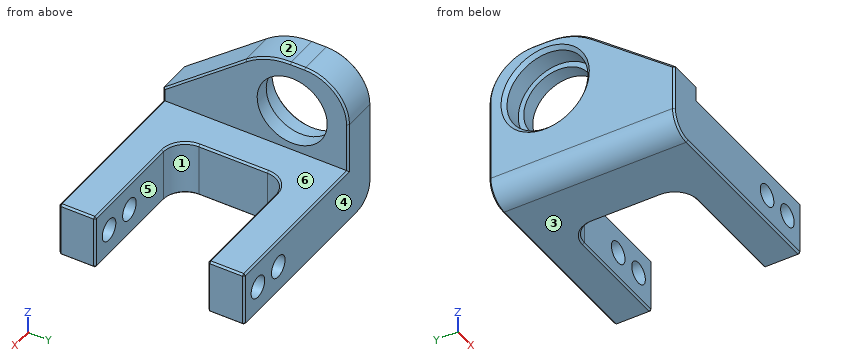
```python
from build123d import *

# Parameters (mm, degrees)
BOSS_EXTRUDE1_DEPTH = 50.8
SKETCH2_R           = 11.1
CUT_EXTRUDE1_DEPTH  = 6
SKETCH4_R           = 9.6
CUT_EXTRUDE2_DEPTH  = 79.563869558
SKETCH5_R           = 3
CUT_EXTRUDE3_DEPTH  = 83.512311809
CUT_EXTRUDE4_DEPTH  = 83.512311809
FILLET3_R           = 20
FILLET4_R           = 12
SKETCH8_W           = 36
SKETCH8_H           = 30.8
CUT_EXTRUDE5_DEPTH  = 80.805586271
CHAMFER2_SIZE       = 1
FILLET6_R           = 6
FILLET5_R           = 6
CHAMFER3_SIZE       = 0.5


with BuildPart() as part:
    # Sketch1 → Boss-Extrude1 (new body)
    with BuildSketch(Plane(origin=(0, 0, 0), x_dir=(1, 0, 0), z_dir=(0, 1, 0))):
        Polygon((-56, 7.5), (-56, -33.04), (-46, -33.04), (-46, -7.5), (0, -7.5), (0, 7.5), align=None)
    extrude(amount=BOSS_EXTRUDE1_DEPTH)

    # Sketch2 → Cut-Extrude1 (cut)
    with BuildSketch(Plane.ZY.offset(56)):
        with Locations((19.04, 35.4)):
            Circle(SKETCH2_R)
    extrude(amount=-CUT_EXTRUDE1_DEPTH, mode=Mode.SUBTRACT)

    # Sketch4 → Cut-Extrude2 (cut, through all)
    with BuildSketch(Plane.ZY.offset(50)):
        with Locations((19.04, 35.4)):
            Circle(SKETCH4_R)
    extrude(amount=-CUT_EXTRUDE2_DEPTH, mode=Mode.SUBTRACT)

    # Sketch5 → Cut-Extrude3 (cut, through all)
    with BuildSketch(Plane(origin=(0, 50.8, 0), x_dir=(1, 0, 0), z_dir=(0, 1, 0))):
        with Locations(Location((-6, 0, 0), (0, 0, 270))):
            Circle(SKETCH5_R)
        with Locations(Location((-15, 0, 0), (0, 0, 270))):
            Circle(SKETCH5_R)
    extrude(amount=-CUT_EXTRUDE3_DEPTH, mode=Mode.SUBTRACT)

    # Sketch6 → Cut-Extrude4 (cut, through all)
    with BuildSketch(Plane.ZY.offset(56)):
        Polygon((11.04, 0), (33.04, 0), (33.04, 28), align=None)
    extrude(amount=-CUT_EXTRUDE4_DEPTH, mode=Mode.SUBTRACT)

    # Fillet3
    fillet3_edges = [part.edges().sort_by_distance(p)[0] for p in [
        (-51, 28, 33.04),
    ]]
    fillet(fillet3_edges, radius=FILLET3_R)

    # Fillet4
    fillet4_edges = [part.edges().sort_by_distance(p)[0] for p in [
        (-51, 50.8, 33.04),
    ]]
    fillet(fillet4_edges, radius=FILLET4_R)

    # Sketch8 → Cut-Extrude5 (cut, through all)
    with BuildSketch(Plane.XY.offset(7.5)):
        with Locations((-18, 25.4)):
            Rectangle(SKETCH8_W, SKETCH8_H)
    extrude(amount=-CUT_EXTRUDE5_DEPTH, mode=Mode.SUBTRACT)

    # Chamfer2
    chamfer2_edges = [part.edges().sort_by_distance(p)[0] for p in [
        (-56, 35.4, 7.94),
    ]]
    chamfer(chamfer2_edges, length=CHAMFER2_SIZE)

    # Fillet6
    fillet6_edges = [part.edges().sort_by_distance(p)[0] for p in [
        (-56, 25.4, -7.5),
    ]]
    fillet(fillet6_edges, radius=FILLET6_R)

    # Fillet5
    fillet5_edges = [part.edges().sort_by_distance(p)[0] for p in [
        (-36, 40.8, 0),
        (-36, 10, 0),
    ]]
    fillet(fillet5_edges, radius=FILLET5_R)

    # Chamfer3
    chamfer3_edges = [part.edges().sort_by_distance(p)[0] for p in [
        (-54.242640687, 50.8, -5.742640687),
        (-15, 10, 7.5),
        (-15, 10, -7.5),
        (-36, 25.4, 7.5),
        (-36, 25.4, -7.5),
        (-34.242640687, 11.757359313, 7.5),
        (-34.242640687, 11.757359313, -7.5),
        (-34.242640687, 39.042640687, 7.5),
        (0, 45.8, 7.5),
        (-34.242640687, 39.042640687, -7.5),
        (0, 45.8, -7.5),
        (-46, 50.8, 14.27),
        (-23, 50.8, 7.5),
        (-46, 11.280415221, 19.903183388),
        (0, 50.8, 0),
        (-56, 11.280415221, 19.903183388),
        (-56, 28.37995835, 31.941419729),
        (-46, 28.37995835, 31.941419729),
        (-46, 36.858630741, 33.04),
        (-46, 47.285281374, 29.525281374),
        (-56, 36.858630741, 33.04),
        (-56, 47.285281374, 29.525281374),
        (-23, 0, 7.5),
        (-46, 0, 9.27),
        (0, 5, 7.5),
        (0, 5, -7.5),
        (0, 10, 0),
        (-15, 40.8, -7.5),
        (0, 40.8, 0),
        (-15, 40.8, 7.5),
        (-25, 0, -7.5),
        (0, 0, 0),
        (-25, 50.8, -7.5),
        (-56, 50.8, 9.77),
        (-56, 0, 4.77),
        (-54.242640687, 0, -5.742640687),
    ]]
    chamfer(chamfer3_edges, length=CHAMFER3_SIZE)


solid = part.part
```
Read the model definition and answer for the solid it produces. Units are mm, in the model's axes. Face numbers are marked on the shaded views. A direction names the side the tool comes from. Give positions to 0.01 mm unless a question says otherwise; leave off trailing zeros. Write each loop counter-clockwise with the first axis right and the second up, starting at its lowest first coordinate (ties: lowest second). Pieces come first, ordered by that corner, then holes. Notation, with made-up numbers: (-17.5, 67) -> (29.5, 67) arc R24 ccw to (29.5, 96) -> close; hole circle Ø2 at (83.25, -31). An arc over 180 degrees is marked (long way). Answer in a Markdown table with one row per item.
1) Each of these flat-tipped pins is pushed along its axis until it touches: pin 1 Ø12.5 at (y, z) = (18.5, 16) entering from +X; pin 2 Ø6 at (x, z) = (-48.5, 16.5) entering from -Y; pin 3 Ø13.5 at (x, y) = (-29, 15) entering from +Z. Where does it stop, or does it pass through?
Results list:
| item | result |
|---|---|
| pin 1 | x = -46 |
| pin 2 | y = 3.13 |
| pin 3 | z = 7.5 |
2) Determine the mould class of the marked faces 1, 2 and 3 for opening direction Y: released by +Y, released by -Y, zero draft, split by the parting line, or undercut.
Results list:
| item | result |
|---|---|
| face 1 | undercut |
| face 2 | released by -Y |
| face 3 | zero draft |
3) Straight lines are drawn through the part: line 1 (X direction, y = 46, z = 0); line 2 (Y direction, x = -3.5, z = 3.5); line 3 (X direction, y = 44.5, z = 23.5). For each, find the intervals that lie inside material, in ascending order. Write a range as [from, to].
Results list:
| item | result |
|---|---|
| line 1 | [-56, -18], [-12, -9], [-3, 0] |
| line 2 | [0, 10], [40.8, 50.8] |
| line 3 | [-50, -46] |
4) Section A-A on x = -15 is taken. Give the vertices of the cut face in (y, z), plus the area to 3 significant figures.
Results list:
| item | result |
|---|---|
| outline | (0, -7) -> (0.5, -7.5) -> (9.5, -7.5) -> (10, -7) -> (10, -3) -> (0, -3) -> close; (0, 3) -> (10, 3) -> (10, 7) -> (9.5, 7.5) -> (0.5, 7.5) -> (0, 7) -> close; (40.8, -7) -> (41.3, -7.5) -> (50.3, -7.5) -> (50.8, -7) -> (50.8, -3) -> (40.8, -3) -> close; (40.8, 3) -> (50.8, 3) -> (50.8, 7) -> (50.3, 7.5) -> (41.3, 7.5) -> (40.8, 7) -> close |
| area | 179 mm^2 |
5) A tool of negligible diameter and unlimited length cuts with its end or side. For the marked faces 4, 5 and 6, from which of +Z, -Z, +X, -X, +Y, -Y can it reach the whole face along a straight path? Write none if from no direction.
Results list:
| item | result |
|---|---|
| face 4 | +Z, -Z, +X, -X, +Y |
| face 5 | +Z, -Z, +X |
| face 6 | +Z, +X, +Y, -Y |
6) Section B-B on z = 19.04 is taken. Give the vertices of the cut face in (x, y), plus the area to 3 significant figures.
Results list:
| item | result |
|---|---|
| outline | (-56, 10.99) -> (-55.5, 10.18) -> (-46.5, 10.18) -> (-46, 10.99) -> (-46, 25.8) -> (-50, 25.8) -> (-50, 24.3) -> (-55, 24.3) -> (-56, 23.3) -> close; (-56, 47.5) -> (-55, 46.5) -> (-50, 46.5) -> (-50, 45) -> (-46, 45) -> (-46, 50.3) -> (-46.5, 50.8) -> (-55.5, 50.8) -> (-56, 50.3) -> close |
| area | 195 mm^2 |
7) Section C-C on x = -47.5 is taken. Give the vertices of the cut face in (y, z), plus the area to 3 significant figures.
Results list:
| item | result |
|---|---|
| outline | (0, -7) -> (0.5, -7.5) -> (50.3, -7.5) -> (50.8, -7) -> (50.8, 21.04) arc R12 ccw to (38.8, 33.04) -> (34.92, 33.04) arc R20 ccw to (22.56, 28.77) -> (0, 11.04) -> close; hole circle Ø19.2 at (35.4, 19.04) |
| area | 1,430 mm^2 |
8) Section D-D on z = 4.5 is taken. Give the vertices of the cut face in (x, y).
Results list:
| item | result |
|---|---|
| outline | (-56, 0.5) -> (-55.5, 0) -> (-0.5, 0) -> (0, 0.5) -> (0, 9.5) -> (-0.5, 10) -> (-30, 10) arc R6 cw to (-36, 16) -> (-36, 34.8) arc R6 cw to (-30, 40.8) -> (-0.5, 40.8) -> (0, 41.3) -> (0, 50.3) -> (-0.5, 50.8) -> (-55.5, 50.8) -> (-56, 50.3) -> close |
